```python
from build123d import *

# Parameters (mm, degrees)
F0_R            = 24.257
F1_DEPTH        = 4.318
F2_R            = 27.94
F2_R_2          = 23.876
F3_DEPTH        = 17.78
F0_W            = 59.944
F0_H            = 59.944
F0_W_2          = 6.35
F0_H_2          = 6.35
F5_DEPTH        = 2.54
F6_DEPTH        = 11.684
F7_D            = 2.54
F8_SIZE         = 2.54
F9_R            = 0.508
F11_D           = 3.175
F11_CSINK_D     = 6.858
F11_CSINK_ANGLE = 90
F12_D           = 5


with BuildPart() as f1:
    # F0 (on Front) → F1 (new body)
    with BuildSketch(Plane.XZ):
        Circle(F0_R)
    extrude(amount=F1_DEPTH)

    # F2 (on Front) → F3 (join)
    with BuildSketch(Plane.XZ):
        Circle(F2_R)
        Circle(F2_R_2, mode=Mode.SUBTRACT)
    extrude(amount=F3_DEPTH)

    # F0 (on Front) → F5 (join)
    with BuildSketch(Plane.XZ):
        Rectangle(F0_W, F0_H)
        with Locations((-23.3818002729, -23.495)):
            Rectangle(F0_W_2, F0_H_2, mode=Mode.SUBTRACT)
        Circle(F0_R, mode=Mode.SUBTRACT)
        with Locations((23.6081997271, -23.495)):
            Rectangle(F0_W_2, F0_H_2, mode=Mode.SUBTRACT)
        with Locations((-23.3818002729, 23.495)):
            Rectangle(F0_W_2, F0_H_2, mode=Mode.SUBTRACT)
        with Locations((23.6081997271, 23.2674991059)):
            Rectangle(F0_W_2, F0_H_2, mode=Mode.SUBTRACT)
    extrude(amount=F5_DEPTH)

    # F0 (on Front) → F6 (join)
    with BuildSketch(Plane.XZ):
        with Locations((-23.3818002729, -23.495)):
            Rectangle(F0_W_2, F0_H_2)
        with Locations((-23.3818002729, 23.495)):
            Rectangle(F0_W_2, F0_H_2)
        with Locations((23.6081997271, 23.2674991059)):
            Rectangle(F0_W_2, F0_H_2)
        with Locations((23.6081997271, -23.495)):
            Rectangle(F0_W_2, F0_H_2)
    extrude(amount=F6_DEPTH)

    # F7 (through all)
    with Locations(Plane(origin=(0, 0, 0), x_dir=(1, 0, 0), z_dir=(0, 1, 0))):
        with Locations((-23.3818002729, -23.495), (23.6081997271, -23.2674991059), (-23.3818002729, 23.495), (23.6081997271, 23.495)):
            Hole(F7_D / 2)

    # F8
    f8_edges = [f1.edges().sort_by_distance(p)[0] for p in [
        (-23.876, -17.78, 0),
    ]]
    chamfer(f8_edges, length=F8_SIZE)

    # F9
    f9_edges = [f1.edges().sort_by_distance(p)[0] for p in [
        (-27.94, -17.78, 0),
    ]]
    fillet(f9_edges, radius=F9_R)

    # F11 (through all)
    with Locations(Plane.XZ.offset(4.318)):
        with Locations((-13.5, -8.257), (13.5, -8.257)):
            CounterSinkHole(F11_D / 2, F11_CSINK_D / 2, counter_sink_angle=F11_CSINK_ANGLE)

    # F12 (through all)
    with Locations(Plane.XZ.offset(4.318)):
        with Locations((0, -14.257)):
            Hole(F12_D / 2)


solid = f1.part
```
Part model, mm, in its own coordinate system. A direction names the side the tool comes from. Coordinates: 2 decimals unless noted, no trailing zeros. Loops run counter-clockwise (first coordinate to the right, second up) from the corner with the lowest first, then second, coordinate; pieces in that order, holes last. Notation, with made-up numbers: (31, 76) - (75, 76) arc R26 cw to (75, 93) - close; hole circle Ø10 at (-22.75, 57.25). An arc over 180 degrees is marked (long way). Write item = value, one per line. Start each with the question number.
Item 1: Flat gauge pins, fed straight in: pin 1 Ø12 at (x, z) = (1.5, -5.5) entering from -Y; pin 2 Ø8 at (x, y) = (8, -14) entering from -Z; pin 3 Ø2.5 at (x, z) = (-13.5, -8.257) entering from +Y; pin 4 Ø7 at (x, y) = (-22, -8) entering from +Z. Where does each tip first touch, or does it go through?
Item 2: Cut at A-A, the plane x = 0. Give the cut face in (y, z), and give its area (3 significant figures).
Item 3: Mould opens along X. For faces 1 (the cylindrical face through (24.5, -5.9, -24.4)), 2 (the flat face through (-23, -7, -20.32)), 3 (the flat face through (-29.972, -1, 0)) say: released by +X, released by -X, zero draft, split by the parting line, or undercut.
Item 4: 3-axis set-ups, long thin cutter, end or side, ignore diameter. For faces 4 (the flat face through (20.433, -7, -24)), 5 (the flat face through (-23, -7, -26.67)), 6 (the flat face through (24, -7, 26.442)): which of +Z, -Z, +X, -X, +Y, -Y reach the whole face in a straight line?
Item 5: Cut at B-B, the plane z = 0. Give the cut face in (x, y), and give its area (3 significant figures).
Item 6: Wall check: L1, parallel to Z at x = 0, y = -1.8; L2, parallel to Z at x = 0, y = -2.7; L3, parallel to Y at x = -27, z = -9.5. Give the ranges that are in metal, low to high. Write a range as from..to.
Item 7: Cut at C-C, the plane y = -12.75. Give the cut face in (x, z), and give its area (3 significant figures).
The answers:
q1.pin_1 = -4.32
q1.pin_2 = -27.65
q1.pin_3 = through
q1.pin_4 = 26.67
q2.outline = (-17.78, -27.43) arc R0.51 ccw to (-17.27, -27.94) - (-2.54, -27.94) - (-2.54, -29.97) - (0, -29.97) - (0, -16.76) - (-4.32, -16.76) - (-4.32, -23.88) - (-15.24, -23.88) - (-17.78, -26.42) - close; (-17.78, 26.42) - (-15.24, 23.88) - (-4.32, 23.88) - (-4.32, -11.76) - (0, -11.76) - (0, 29.97) - (-2.54, 29.97) - (-2.54, 27.94) - (-17.27, 27.94) arc R0.51 ccw to (-17.78, 27.43) - close
q2.area = 333 mm2
q3.face_1 = undercut
q3.face_2 = zero draft
q3.face_3 = released by -X
q4.face_4 = -Z, -Y
q4.face_5 = -Z, -X, -Y
q4.face_6 = +Z, +X, -Y
q5.outline = (-29.97, -2.54) - (-27.94, -2.54) - (-27.94, -17.27) arc R0.51 ccw to (-27.43, -17.78) - (-26.42, -17.78) - (-23.88, -15.24) - (-23.88, -4.32) - (23.88, -4.32) - (23.88, -15.24) - (26.42, -17.78) - (27.43, -17.78) arc R0.51 ccw to (27.94, -17.27) - (27.94, -2.54) - (29.97, -2.54) - (29.97, 0) - (-29.97, 0) - close
q5.area = 354 mm2
q6.L1 = -29.97..-16.76, -11.76..29.97
q6.L2 = -27.94..-16.76, -11.76..27.94
q6.L3 = -2.54..0
q7.outline = circle Ø55.88 at (0, 0); hole circle Ø47.75 at (0, 0)
q7.area = 662 mm2
